Source: CAD feature listing. Evaluate the final solid. Frame: model axes, mm. Face numbers are marked on the shaded views. A direction names the side the tool comes from. Round coordinates to 2 decimals unless told otherwise and drop trailing zeros. Order: outer loops, then holes, each group sorted by start corner. A loop starts at its lowest first (then second) coordinate and runs counter-clockwise, first axis right, second up. Notation, with made-up numbers: (56.25, 4.25) -> (102.25, 4.25) arc R6 cw to (102.25, 12.25) -> close; hole circle Ø3 at (-13.75, 63). An arc over 180 degrees is marked (long way). Write item = value, one per line. Start each with the question number.
(1) Cut plane C-C on y = 21.5. Return the cut outline in (x, z).
(2) Reachability of the marked faces 5, 6 and 7 from +Z, -Z, +X, -X, +Y, -Y: full face, straight path, thin tool, end or side. Return the list, or none.
(3) Cut plane D-D on x = 59.5. Return the cut outline in (y, z).
(4) Contact query for flat-ended pins moving along their axis: pin 1 Ø7 at (y, z) = (51.5, 11) entering from +X; pin 2 Ø0.7 at (x, z) = (-22, 10) entering from +Y; pin 3 Ø4 at (x, z) = (-10, 12) entering from +Y; pin 4 Ø2 at (y, z) = (7.5, 6) entering from +X. Output: stop coordinate, or through.
(5) Draft query along Z for the marked faces 1, 2, 3 and 4. Return one class per face: released by +Z, released by -Z, zero draft, split by the parting line, or undercut.
(6) Cut plane A-A on x = -3.5. Return the cut outline in (y, z), then the cut area to 3 significant figures.
(7) Cut plane B-B on z = 6.5. Give the number of separate pieces and of enclosed holes in the cut face, then the cut area to 3 significant figures.
(8) Ray query, line 1 (X direction, y = 49.5, z = 8.5); line 2 (Z direction, x = 37, y = 47); line 3 (X direction, y = 60.5, z = 11.25). Return the intervals inside material, ascending.
from build123d import *

# Parameters (mm, degrees)
BOX006_W               = 21
BOX006_H               = 36
BOX006_DEPTH           = 10
CYLINDER013_R          = 1.1
CYLINDER013_DEPTH      = 10
CYLINDER014_R          = 1.1
CYLINDER014_DEPTH      = 10
SKETCH019_W            = 23.3
SKETCH019_H            = 12.5
PAD019_DEPTH           = 19.5
SKETCH017_W            = 32.5
SKETCH017_H            = 12.5
PAD018_DEPTH           = 4.5
SKETCH018_W            = 36.061928
SKETCH018_H            = 25.639376
PAD017_DEPTH           = 14
CYLINDER015_R          = 1.1
CYLINDER015_DEPTH      = 10
CYLINDER016_R          = 1.1
CYLINDER016_DEPTH      = 10
SKETCH022_W            = 23.3
SKETCH022_H            = 12.5
PAD022_DEPTH           = 19.5
SKETCH020_W            = 32.5
SKETCH020_H            = 12.5
PAD021_DEPTH           = 4.5
SKETCH021_W            = 36.061928
SKETCH021_H            = 25.639376
PAD020_DEPTH           = 14
CUT019_PLACEMENT_ANGLE = 180
CYLINDER017_R          = 1.1
CYLINDER017_DEPTH      = 10
CYLINDER018_R          = 1.1
CYLINDER018_DEPTH      = 10
SKETCH025_W            = 23.3
SKETCH025_H            = 12.5
PAD025_DEPTH           = 19.5
SKETCH023_W            = 32.5
SKETCH023_H            = 12.5
PAD024_DEPTH           = 4.5
SKETCH024_W            = 36.061928
SKETCH024_H            = 25.639376
PAD023_DEPTH           = 14
CUT022_PLACEMENT_ANGLE = 180
PAD016_DEPTH           = 2.5


with BuildPart() as cube006:
    # Box006 → Box006 (new body)
    with BuildSketch(Plane(origin=(-10.5, -34, 0), x_dir=(1, 0, 0), z_dir=(0, 0, 1))):
        with Locations((10.5, 18)):
            Rectangle(BOX006_W, BOX006_H)
    extrude(amount=BOX006_DEPTH)


with BuildPart() as cylinder013:
    # Cylinder013 → Cylinder013 (new body)
    with BuildSketch(Plane(origin=(30, 22, 6), x_dir=(1, 0, 0), z_dir=(0, -1, 0))):
        Circle(CYLINDER013_R)
    extrude(amount=CYLINDER013_DEPTH)


with BuildPart() as obj1:
    # Cylinder014 → Cylinder014 (new body)
    with BuildSketch(Plane(origin=(2.2, 22, 6), x_dir=(1, 0, 0), z_dir=(0, -1, 0))):
        Circle(CYLINDER014_R)
    extrude(amount=CYLINDER014_DEPTH)

    # Fusion014: union Cylinder013
    add(cylinder013.part)


with BuildPart() as cortecuerpo002:
    # Sketch019 → Pad019 (new body)
    with BuildSketch(Plane.XZ):
        with Locations((16.4, 6.25)):
            Rectangle(SKETCH019_W, SKETCH019_H)
    extrude(amount=PAD019_DEPTH)


with BuildPart() as cortecuerpo002_1:
    # Body021 placement: moved
    add(cortecuerpo002.part.moved(Location((0, 19, 0))))


with BuildPart() as cortetornillos002:
    # Sketch017 → Pad018 (new body)
    with BuildSketch(Plane.XZ):
        with Locations((16.25, 6.25)):
            Rectangle(SKETCH017_W, SKETCH017_H)
    extrude(amount=PAD018_DEPTH)


with BuildPart() as cortetornillos002_1:
    # Body020 placement: moved
    add(cortetornillos002.part.moved(Location((0, 23, 0))))


with BuildPart() as obj2:
    # Sketch018 → Pad017 (new body)
    with BuildSketch(Plane.XY):
        with Locations((15.881367, 9.413649)):
            Rectangle(SKETCH018_W, SKETCH018_H)
    extrude(amount=PAD017_DEPTH)


with BuildPart() as obj2_1:
    # Body019 placement: moved
    add(obj2.part.moved(Location((0, 0, -1))))

    # Cut014: cut CorteTornillos002
    add(cortetornillos002_1.part, mode=Mode.SUBTRACT)

    # Cut015: cut CorteCuerpo002
    add(cortecuerpo002_1.part, mode=Mode.SUBTRACT)

    # Cut016: cut obj1
    add(obj1.part, mode=Mode.SUBTRACT)


with BuildPart() as obj2_2:
    # Cut016 placement: moved
    add(obj2_1.part.moved(Location((-24, 39, 4))))


with BuildPart() as cylinder015:
    # Cylinder015 → Cylinder015 (new body)
    with BuildSketch(Plane(origin=(30, 22, 6), x_dir=(1, 0, 0), z_dir=(0, -1, 0))):
        Circle(CYLINDER015_R)
    extrude(amount=CYLINDER015_DEPTH)


with BuildPart() as obj3:
    # Cylinder016 → Cylinder016 (new body)
    with BuildSketch(Plane(origin=(2.2, 22, 6), x_dir=(1, 0, 0), z_dir=(0, -1, 0))):
        Circle(CYLINDER016_R)
    extrude(amount=CYLINDER016_DEPTH)

    # Fusion015: union Cylinder015
    add(cylinder015.part)


with BuildPart() as cortecuerpo003:
    # Sketch022 → Pad022 (new body)
    with BuildSketch(Plane.XZ):
        with Locations((16.4, 6.25)):
            Rectangle(SKETCH022_W, SKETCH022_H)
    extrude(amount=PAD022_DEPTH)


with BuildPart() as cortecuerpo003_1:
    # Body024 placement: moved
    add(cortecuerpo003.part.moved(Location((0, 19, 0))))


with BuildPart() as cortetornillos003:
    # Sketch020 → Pad021 (new body)
    with BuildSketch(Plane.XZ):
        with Locations((16.25, 6.25)):
            Rectangle(SKETCH020_W, SKETCH020_H)
    extrude(amount=PAD021_DEPTH)


with BuildPart() as cortetornillos003_1:
    # Body023 placement: moved
    add(cortetornillos003.part.moved(Location((0, 23, 0))))


with BuildPart() as obj4:
    # Sketch021 → Pad020 (new body)
    with BuildSketch(Plane.XY):
        with Locations((15.881367, 9.413649)):
            Rectangle(SKETCH021_W, SKETCH021_H)
    extrude(amount=PAD020_DEPTH)


with BuildPart() as obj4_1:
    # Body022 placement: moved
    add(obj4.part.moved(Location((0, 0, -1))))

    # Cut017: cut CorteTornillos003
    add(cortetornillos003_1.part, mode=Mode.SUBTRACT)

    # Cut018: cut CorteCuerpo003
    add(cortecuerpo003_1.part, mode=Mode.SUBTRACT)

    # Cut019: cut obj3
    add(obj3.part, mode=Mode.SUBTRACT)


with BuildPart() as obj4_2:
    # Cut019 placement: moved
    add(obj4_1.part.moved(Location((-67, 62, 16.5))).rotate(Axis((-67, 62, 16.5), (1, 0, 0)), CUT019_PLACEMENT_ANGLE))


with BuildPart() as cylinder017:
    # Cylinder017 → Cylinder017 (new body)
    with BuildSketch(Plane(origin=(30, 22, 6), x_dir=(1, 0, 0), z_dir=(0, -1, 0))):
        Circle(CYLINDER017_R)
    extrude(amount=CYLINDER017_DEPTH)


with BuildPart() as obj5:
    # Cylinder018 → Cylinder018 (new body)
    with BuildSketch(Plane(origin=(2.2, 22, 6), x_dir=(1, 0, 0), z_dir=(0, -1, 0))):
        Circle(CYLINDER018_R)
    extrude(amount=CYLINDER018_DEPTH)

    # Fusion016: union Cylinder017
    add(cylinder017.part)


with BuildPart() as cortecuerpo004:
    # Sketch025 → Pad025 (new body)
    with BuildSketch(Plane.XZ):
        with Locations((16.4, 6.25)):
            Rectangle(SKETCH025_W, SKETCH025_H)
    extrude(amount=PAD025_DEPTH)


with BuildPart() as cortecuerpo004_1:
    # Body027 placement: moved
    add(cortecuerpo004.part.moved(Location((0, 19, 0))))


with BuildPart() as cortetornillos004:
    # Sketch023 → Pad024 (new body)
    with BuildSketch(Plane.XZ):
        with Locations((16.25, 6.25)):
            Rectangle(SKETCH023_W, SKETCH023_H)
    extrude(amount=PAD024_DEPTH)


with BuildPart() as cortetornillos004_1:
    # Body026 placement: moved
    add(cortetornillos004.part.moved(Location((0, 23, 0))))


with BuildPart() as obj6:
    # Sketch024 → Pad023 (new body)
    with BuildSketch(Plane.XY):
        with Locations((15.881367, 9.413649)):
            Rectangle(SKETCH024_W, SKETCH024_H)
    extrude(amount=PAD023_DEPTH)


with BuildPart() as obj6_1:
    # Body025 placement: moved
    add(obj6.part.moved(Location((0, 0, -1))))

    # Cut020: cut CorteTornillos004
    add(cortetornillos004_1.part, mode=Mode.SUBTRACT)

    # Cut021: cut CorteCuerpo004
    add(cortecuerpo004_1.part, mode=Mode.SUBTRACT)

    # Cut022: cut obj5
    add(obj5.part, mode=Mode.SUBTRACT)


with BuildPart() as obj6_2:
    # Cut022 placement: moved
    add(obj6_1.part.moved(Location((35, 62, 16.5))).rotate(Axis((35, 62, 16.5), (1, 0, 0)), CUT022_PLACEMENT_ANGLE))


with BuildPart() as cut031:
    # Sketch016 → Pad016 (new body)
    with BuildSketch(Plane.XY):
        Polygon((-72.5, 36), (-72.5, 66), (72.5, 66), (72.5, 36), (37.5, 36), (37.5, -34), (-37.5, -34), (-37.5, 36), align=None)
    extrude(amount=PAD016_DEPTH)


with BuildPart() as cut031_1:
    # Body018 placement: moved
    add(cut031.part.moved(Location((0, 0, 1))))

    # Fusion022: union obj2, obj4, obj6
    add(obj2_2.part)
    add(obj4_2.part)
    add(obj6_2.part)

    # Cut031: cut Cube006
    add(cube006.part, mode=Mode.SUBTRACT)


solid = cut031_1.part
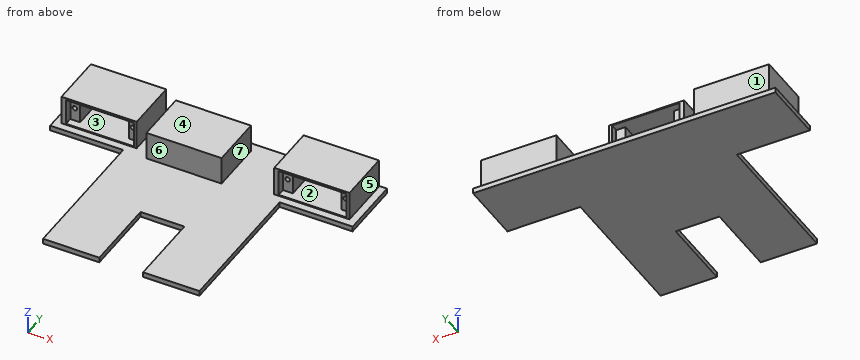
Evaluation:
q1.outline = (-37.5, 1) -> (37.5, 1) -> (37.5, 3.5) -> (-37.5, 3.5) -> close
q2.face_5 = +Z, +X, +Y, -Y
q2.face_6 = +Z, +X, -X, -Y
q2.face_7 = +Z, +Y, -Y
q3.outline = (36, 1) -> (66, 1) -> (66, 3.5) -> (65.41, 3.5) -> (65.41, 17.5) -> (39.77, 17.5) -> (39.77, 16.5) -> (62.5, 16.5) -> (62.5, 4) -> (39.77, 4) -> (39.77, 3.5) -> (36, 3.5) -> close
q4.pin_1 = 68.91
q4.pin_2 = 51
q4.pin_3 = 38.5
q4.pin_4 = through
q5.face_1 = zero draft
q5.face_2 = undercut
q5.face_3 = undercut
q5.face_4 = released by +Z
q6.outline = (2, 1) -> (66, 1) -> (66, 3.5) -> (61.23, 3.5) -> (61.23, 4) -> (38.5, 4) -> (38.5, 16.5) -> (61.23, 16.5) -> (61.23, 17) -> (35.59, 17) -> (35.59, 3.5) -> (2, 3.5) -> close
q6.area = 222 mm^2
q7.separate_pieces = 3
q7.enclosed_holes = 0
q7.area = 1,080 mm^2
q8.line_1 = -69.15 to -62.25, -38.95 to -33.09, -26.15 to -19.25, 4.05 to 9.91, 32.85 to 39.75, 63.05 to 68.91
q8.line_2 = 1 to 9.42, 11.58 to 17.5
q8.line_3 = -69.15 to -62.25, -38.95 to -33.09, -26.15 to -24, 8.5 to 9.91, 32.85 to 39.75, 63.05 to 68.91
